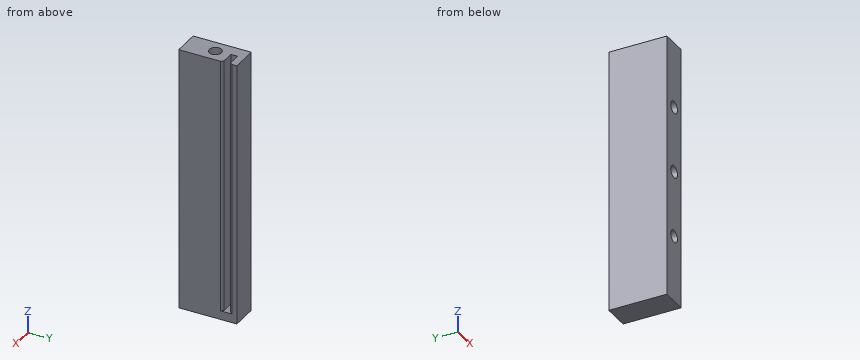
```python
from build123d import *

# Parameters (mm, degrees)
SKETCH_1_W          = 9
SKETCH_1_H          = 15
EXTRUDE_1_DEPTH     = 90
SKETCH_2_R          = 2.1
CUT_EXTRUDE_1_DEPTH = 6
SKETCH_3_W          = 5
SKETCH_3_H          = 2.25
EXTRUDE_2_DEPTH     = 3
CHAMFER_1_SIZE      = 0.75
SKETCH_4_R          = 2.1
CUT_EXTRUDE_2_DEPTH = 6


with BuildPart() as part:
    # Эскиз1 → Бобышка-Вытянуть1 (new body)
    with BuildSketch(Plane.XY):
        Rectangle(SKETCH_1_W, SKETCH_1_H)
        Polygon((-4.5, 12.25), (-4.5, 7.5), (-0.5, 7.5), (-0.5, 9.75), (4.5, 9.75), (4.5, 12.25), align=None)
    extrude(amount=EXTRUDE_1_DEPTH)

    # Эскиз2 → Вырез-Вытянуть1 (cut)
    with BuildSketch(Plane.XZ.offset(7.5)):
        with Locations(Location((0, 22.5, 0), (0, 0, 270))):
            Circle(SKETCH_2_R)
        with Locations(Location((0, 67.5, 0), (0, 0, 270))):
            Circle(SKETCH_2_R)
        with Locations(Location((0, 45, 0), (0, 0, 270))):
            Circle(SKETCH_2_R)
    extrude(amount=-CUT_EXTRUDE_1_DEPTH, mode=Mode.SUBTRACT)

    # Эскиз3 → Бобышка-Вытянуть2 (add)
    with BuildSketch(Plane(origin=(0, 0, 0), x_dir=(-1, 0, 0), z_dir=(0, 0, -1))):
        with Locations((-2, 8.625)):
            Rectangle(SKETCH_3_W, SKETCH_3_H)
    extrude(amount=-EXTRUDE_2_DEPTH)

    # Фаска1
    chamfer_1_edges = [part.edges().sort_by_distance(p)[0] for p in [
        (4.5, 9.75, 46.5),
        (4.5, 7.5, 46.5),
    ]]
    chamfer(chamfer_1_edges, length=CHAMFER_1_SIZE)

    # Эскиз4 → Вырез-Вытянуть2 (cut)
    with BuildSketch(Plane.XY.offset(90)):
        with Locations((0, 2.5)):
            Circle(SKETCH_4_R)
    extrude(amount=-CUT_EXTRUDE_2_DEPTH, mode=Mode.SUBTRACT)


solid = part.part
```
Geometry check sheet. Reference: the model listing, model coordinates, mm. Coordinates: 2 decimals unless noted, no trailing zeros. Write each loop counter-clockwise with the first axis right and the second up, starting at its lowest first coordinate (ties: lowest second). Pieces come first, ordered by that corner, then holes. Notation, with made-up numbers: M 19,89.25 L 32,89.25 A22 cw 32,125.25 Z; hole C -19.5,-40 d8. An arc over 180 degrees is marked long. One line per item, written item: value. Start each with the question number.
(1) Scan lines: line 1 along Y through (x, z) = (0, 87.75); line 2 along Y through (x, z) = (1.25, 6.5); line 3 along Z through (x, y) = (1.75, 9). Record each from-to range of solid material in increasing order. Write a range as [from, to].
(2) Sectioned sample at B-B, the plane y = 2.5. Enter the section's corners in (x, z), and give its area (3 significant figures).
(3) Sectioned sample at A-A, the plane z = 28.5. Enter the section's corners in (x, y), and give its area (3 significant figures).
(4) Depth check by flat-ended pin: pin 1 (2 mm diameter, centred on y = 9, z = 47.5, fed in from +X); pin 2 (1.3 mm diameter, centred on x = 1, z = 44, fed in from -Y); pin 3 (2 mm diameter, centred on x = 0, y = 2, fed in from +Z). Enter the tip coordinate at first touch or a pass-through.
(5) Sectioned sample at C-C, the plane z = 45. Enter the section's corners in (x, y).
Filled sheet:
1. line 1: [-7.5, 0.4], [4.6, 7.5], [9.75, 12.25]
1. line 2: [-7.5, 7.5], [9.75, 12.25]
1. line 3: [0, 3]
2. outline: M -4.5,0 L 4.5,0 L 4.5,90 L 2.1,90 L 2.1,84 L -2.1,84 L -2.1,90 L -4.5,90 Z
2. area: 785 mm²
3. outline: M -4.5,-7.5 L 4.5,-7.5 L 4.5,6.75 L 3.75,7.5 L -0.5,7.5 L -0.5,9.75 L 3.75,9.75 L 4.5,10.5 L 4.5,12.25 L -4.5,12.25 Z
3. area: 166 mm²
4. pin 1: x = 4
4. pin 2: y = -1.5
4. pin 3: z = 84
5. outline: M -4.5,-7.5 L -2.1,-7.5 L -2.1,-1.5 L 2.1,-1.5 L 2.1,-7.5 L 4.5,-7.5 L 4.5,6.75 L 3.75,7.5 L -0.5,7.5 L -0.5,9.75 L 3.75,9.75 L 4.5,10.5 L 4.5,12.25 L -4.5,12.25 Z
